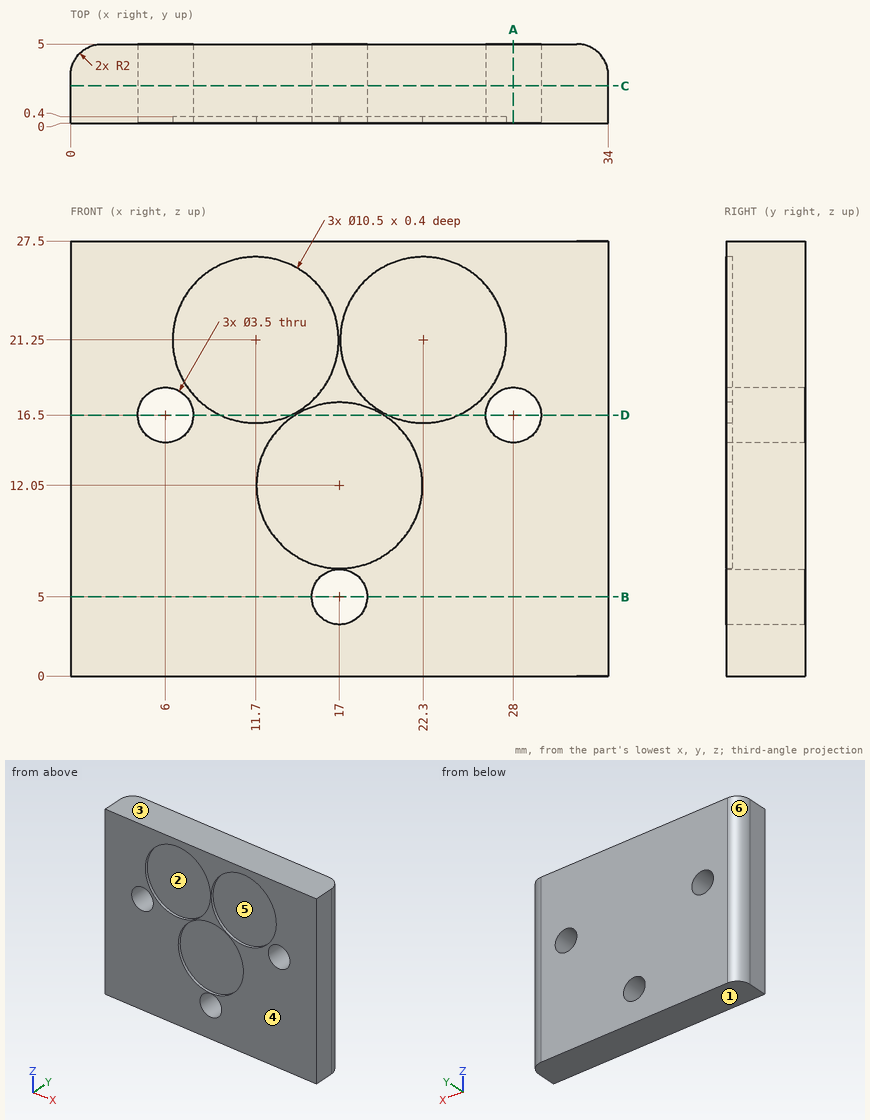
Study the drawing (mm; zero at the part's minimum x, y, z) and answer. A direction names the side the tool comes from. Coordinates: 2 decimals unless noted, no trailing zeros. Loops run counter-clockwise (first coordinate to the right, second up) from the corner with the lowest first, then second, coordinate; pieces in that order, holes last. Notation, with made-up numbers: M -8,76 L 50,76 A34 ccw 50,106 Z; hole C -0.75,76 d8. An arc over 180 degrees is marked long. Answer in a Markdown table with one row per item.
1) Find section C-C (y = 2.35). Determine the outline of the cut face in (x, z).
Answers below:
| item | result |
|---|---|
| outline | M 0,0 L 34,0 L 34,27.5 L 0,27.5 Z; hole C 6,16.5 d3.5; hole C 17,5 d3.5; hole C 28,16.5 d3.5 |
2) Determine the mould class of the marked faces 1, 2, 3 and 4 for opening direction Z: released by +Z, released by -Z, zero draft, split by the parting line, or undercut.
Answers below:
| item | result |
|---|---|
| face 1 | released by -Z |
| face 2 | undercut |
| face 3 | released by +Z |
| face 4 | zero draft |
3) Find the intervals of material crossed by probe 1 along X at (y, z) = (1.05, 16.5); probe 2 along X at (y, z) = (3.6, 15); probe 3 along Y at (x, z) = (10.5, 25.75), in increasing order.
Answers below:
| item | result |
|---|---|
| probe 1 | 0 to 4.25, 7.75 to 26.25, 29.75 to 34 |
| probe 2 | 0.09 to 5.1, 6.9 to 27.1, 28.9 to 33.91 |
| probe 3 | 0.4 to 5 |
4) Find section A-A (x = 28). Determine the outline of the cut face in (y, z).
Answers below:
| item | result |
|---|---|
| outline | M 0,0 L 5,0 L 5,14.75 L 0,14.75 Z; M 0,18.25 L 5,18.25 L 5,27.5 L 0,27.5 Z |
5) Given pin 1 (8.5 mm diameter, centred on x = 24, z = 20.5, fed in from -Y); pin 2 (3 mm diameter, centred on x = 17, z = 5, fed in from -Y); pin 3 (3 mm diameter, centred on x = 18.5, z = 11, fed in from -Y); pin 4 (1.5 mm diameter, centred on y = 4.5, z = 3, fed in from +X), each flat-ended and moving along its own axis, determine where each tip first touches the part or whether it passes through.
Answers below:
| item | result |
|---|---|
| pin 1 | y = 0 |
| pin 2 | through |
| pin 3 | y = 0.4 |
| pin 4 | x = 33.85 |
6) Find section D-D (z = 16.5). Determine the outline of the cut face in (x, y).
Answers below:
| item | result |
|---|---|
| outline | M 0,0 L 4.25,0 L 4.25,5 L 2,5 A2 ccw 0,3 Z; M 7.75,0 L 9.46,0 L 9.46,0.4 L 13.94,0.4 L 13.94,0 L 14.21,0 L 14.21,0.4 L 19.79,0.4 L 19.79,0 L 20.06,0 L 20.06,0.4 L 24.54,0.4 L 24.54,0 L 26.25,0 L 26.25,5 L 7.75,5 Z; M 29.75,0 L 34,0 L 34,3 A2 ccw 32,5 L 29.75,5 Z |
7) Find section B-B (z = 5). Determine the outline of the cut face in (x, y).
Answers below:
| item | result |
|---|---|
| outline | M 0,0 L 15.25,0 L 15.25,5 L 2,5 A2 ccw 0,3 Z; M 18.75,0 L 34,0 L 34,3 A2 ccw 32,5 L 18.75,5 Z |
8) Which of the six approach directions +Z, -Z, +X, -X, +Y, -Y give full straight-line access (tool end or side, diameter ignored) to the marked faces 5 and 6?
Answers below:
| item | result |
|---|---|
| face 5 | -Y |
| face 6 | +Z, -Z, -X, +Y |
